Check sheet for the modelled part. Datum: model origin and axes. Units: mm. Face numbers are marked on the shaded views. A direction names the side the tool comes from. Give positions to 0.01 mm unless a question says otherwise; leave off trailing zeros. Order: outer loops, then holes, each group sorted by start corner. A loop starts at its lowest first (then second) coordinate and runs counter-clockwise, first axis right, second up.
```python
from build123d import *

# Parameters (mm, degrees)
F0_R     = 3.175
F0_R_2   = 19.05
F1_DEPTH = 6.35
F2_R     = 31.75
F2_R_2   = 28.575
F3_DEPTH = 44.45
F4_SIZE2 = 1.905
F4_SIZE  = 1.905
F5_R     = 25.4
F5_R_2   = 19.05
F6_DEPTH = 31.75
F7_R     = 2.54


with BuildPart() as f1:
    # F0 (on Right) → F1 (new body)
    with BuildSketch(Plane.YZ):
        with BuildLine():
            ThreePointArc((-38.1, -31.75), (-36.240128, -36.240128), (-31.75, -38.1))
            Line((-31.75, -38.1), (31.75, -38.1))
            ThreePointArc((31.75, -38.1), (36.240128, -36.240128), (38.1, -31.75))
            Line((38.1, -31.75), (38.1, 31.75))
            ThreePointArc((38.1, 31.75), (36.240128, 36.240128), (31.75, 38.1))
            Line((31.75, 38.1), (-31.75, 38.1))
            ThreePointArc((-31.75, 38.1), (-36.240128, 36.240128), (-38.1, 31.75))
            Line((-38.1, 31.75), (-38.1, -31.75))
        make_face()
        with Locations((-31.7495, -31.498018)):
            Circle(F0_R, mode=Mode.SUBTRACT)
        with Locations((31.75, -31.75)):
            Circle(F0_R, mode=Mode.SUBTRACT)
        with Locations((-31.7495, 32.001982)):
            Circle(F0_R, mode=Mode.SUBTRACT)
        Circle(F0_R_2, mode=Mode.SUBTRACT)
        with Locations((31.75, 31.75)):
            Circle(F0_R, mode=Mode.SUBTRACT)
    extrude(amount=F1_DEPTH)

    # F2 (on Right) → F3 (join)
    with BuildSketch(Plane.YZ):
        Circle(F2_R)
        Circle(F2_R_2, mode=Mode.SUBTRACT)
    extrude(amount=F3_DEPTH)

    # F4
    f4_edges = [f1.edges().sort_by_distance(p)[0] for p in [
        (44.45, -31.75, 0),
    ]]
    chamfer(f4_edges, length=F4_SIZE, length2=F4_SIZE2)

    # F5 (on Right) → F6 (join)
    with BuildSketch(Plane.YZ):
        Circle(F5_R)
        Circle(F5_R_2, mode=Mode.SUBTRACT)
    extrude(amount=-F6_DEPTH)

    # F7
    f7_edges = [f1.edges().sort_by_distance(p)[0] for p in [
        (-31.75, -25.4, 0),
    ]]
    fillet(f7_edges, radius=F7_R)


solid = f1.part
```
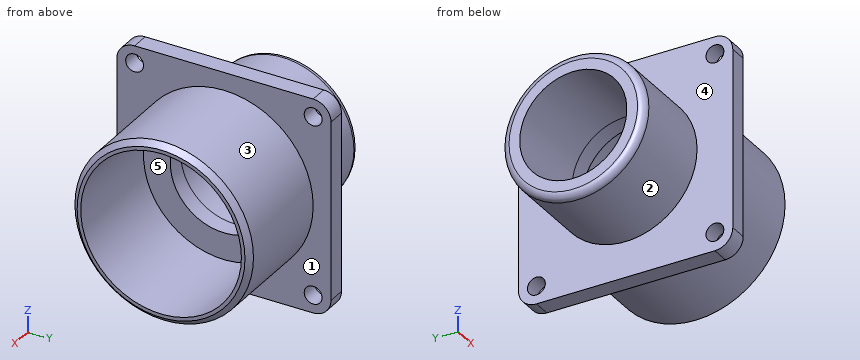
(1) Gauge pin test, flat ends, axial feed: pin 1 Ø5 at (y, z) = (-22, 15) entering from -X; pin 2 Ø8 at (y, z) = (-28.5, -27) entering from +X; pin 3 Ø4 at (x, y) = (-21, 8) entering from -Z. Record the tip position at first contact, or that the pin passes through.
Response values:
pin 1: stops at x = -31.41
pin 2: stops at x = 6.35
pin 3: stops at z = -24.68
(2) Cross-section at A-A on y = 0. Enter the section's corners in (x, z) (3 decimals), then the cut area to 3 significant figures.
Response values:
outline: (-31.75, -22.86) arc R2.54 ccw to (-29.21, -25.4) - (0, -25.4) - (0, -38.1) - (6.35, -38.1) - (6.35, -31.75) - (42.545, -31.75) - (44.45, -29.845) - (44.45, -28.575) - (6.35, -28.575) - (6.35, -19.05) - (-31.75, -19.05) - close; (-31.75, 19.05) - (6.35, 19.05) - (6.35, 28.575) - (44.45, 28.575) - (44.45, 29.845) - (42.545, 31.75) - (6.35, 31.75) - (6.35, 38.1) - (0, 38.1) - (0, 25.4) - (-29.21, 25.4) arc R2.54 ccw to (-31.75, 22.86) - close
area: 881 mm2
(3) Release check for a two-part mould opening along Z. For the marked faces 3, 4 and 5 record: released by +Z, released by -Z, zero draft, split by the parting line, or undercut.
Response values:
face 3: split by the parting line
face 4: zero draft
face 5: undercut
(4) Cross-section at D-D on x = 12. Enter the section's corners in (y, z) (3 decimals).
Response values:
outline: circle Ø63.5 at (0, 0); hole circle Ø57.15 at (0, 0)
(5) Material ranges on L1, parallel to Z at x = 4, y = 31; L2, parallel to Z at x = -17, y = 0; L3, parallel to Y at x = 28.5, z = 0 (3 decimals), recorded low to high.
Response values:
L1: z = -38.1 to -34.84, -28.66 to 28.66, 34.84 to 38.1
L2: z = -25.4 to -19.05, 19.05 to 25.4
L3: y = -31.75 to -28.575, 28.575 to 31.75
(6) Cross-section at C-C on y = 33.5. Enter the section's corners in (x, z), then the cut area to 3 significant figures.
Response values:
outline: (0, -37.85) - (6.35, -37.85) - (6.35, -34.4) - (0, -34.4) - close; (0, -29.1) - (6.35, -29.1) - (6.35, 29.1) - (0, 29.1) - close; (0, 34.4) - (6.35, 34.4) - (6.35, 37.85) - (0, 37.85) - close
area: 413 mm2
(7) Set-up check for the marked faces 1 and 2: record each of +Z, -Z, +X, -X, +Y, -Y from which the full face is reachable in a straight line by a thin tool's end or side.
Response values:
face 1: +X
face 2: -X
